Work out the finished part from the listing and answer in its coordinate system (mm). Round coordinates to 2 decimals unless told otherwise and drop trailing zeros. Loops run counter-clockwise (first coordinate to the right, second up) from the corner with the lowest first, then second, coordinate; pieces in that order, holes last. Notation, with made-up numbers: (61.25, 68.25) - (70.25, 68.25) arc R20 ccw to (70.25, 96.25) - close; hole circle Ø1 at (62.5, -13). An arc over 180 degrees is marked (long way). Answer as CSV lines item,"result". Start each with the question number.
```python
from build123d import *

# Parameters (mm, degrees)
F0_W     = 1016
F0_H     = 1930.4
F1_DEPTH = 50.8
F2_W     = 381
F2_H     = 304.8
F3_DEPTH = 50.801


with BuildPart() as f1:
    # F0 (on Front) → F1 (new body)
    with BuildSketch(Plane.XZ):
        Rectangle(F0_W, F0_H)
    extrude(amount=F1_DEPTH)

    # F2 (on face) → F3 (cut, through all)
    with BuildSketch(Plane.XZ.offset(50.8)):
        with Locations((-215.9, 660.4)):
            Rectangle(F2_W, F2_H)
        with Locations((-215.9, 330.2)):
            Rectangle(F2_W, F2_H)
        with Locations((-215.9, 0)):
            Rectangle(F2_W, F2_H)
        with Locations((-215.9, -330.2)):
            Rectangle(F2_W, F2_H)
        with Locations((-215.9, -660.4)):
            Rectangle(F2_W, F2_H)
        with Locations((215.9, 330.2)):
            Rectangle(F2_W, F2_H)
        with Locations((215.9, 660.4)):
            Rectangle(F2_W, F2_H)
        with Locations((215.9, 0)):
            Rectangle(F2_W, F2_H)
        with Locations((215.9, -330.2)):
            Rectangle(F2_W, F2_H)
        with Locations((215.9, -660.4)):
            Rectangle(F2_W, F2_H)
    extrude(amount=-F3_DEPTH, mode=Mode.SUBTRACT)


solid = f1.part
```
Item 1: Determine the mould class of faces 1 (the face through (-7, -25, 965.2)), 2 (the face through (508, -25, -14)), 3 (the face through (213, -26, -152.4)), 4 (the face through (-508, -25, -14)) for opening direction X: pulls with the +X half, pulls with the -X half, needs draft (parallel to the pull), parting line crosses it, or undercut.
Item 2: Section B-B, the plane x = 361 is taken. Give the vertices of the cut face in (y, z), and give its area (3 significant figures).
Item 3: Find the intervals of material crossed by L1, parallel to Z at x = 128.5, y = -33; L2, parallel to X at y = -12, z = -692, in increasing order.
Item 4: Section C-C, the plane y = -21.5 is taken. Count the separate pieces of the cut face and the enclosed holes in it, and give its area (3 significant figures).
Item 5: Section A-A, the plane z = 375.5 is taken. Give the vertices of the cut face in (x, y).
Answer:
1,face 1,"needs draft"
1,face 2,"pulls with the +X half"
1,face 3,"undercut"
1,face 4,"pulls with the -X half"
2,outline,"(-50.8, -965.2) - (0, -965.2) - (0, -812.8) - (-50.8, -812.8) - close; (-50.8, -508) - (0, -508) - (0, -482.6) - (-50.8, -482.6) - close; (-50.8, -177.8) - (0, -177.8) - (0, -152.4) - (-50.8, -152.4) - close; (-50.8, 152.4) - (0, 152.4) - (0, 177.8) - (-50.8, 177.8) - close; (-50.8, 482.6) - (0, 482.6) - (0, 508) - (-50.8, 508) - close; (-50.8, 812.8) - (0, 812.8) - (0, 965.2) - (-50.8, 965.2) - close"
2,area,"20,600 mm²"
3,L1,"z = -965.2 to -812.8, -508 to -482.6, -177.8 to -152.4, 152.4 to 177.8, 482.6 to 508, 812.8 to 965.2"
3,L2,"x = -508 to -406.4, -25.4 to 25.4, 406.4 to 508"
4,separate pieces,"1"
4,enclosed holes,"10"
4,area,"800,000 mm²"
5,outline,"(-508, -50.8) - (-406.4, -50.8) - (-406.4, 0) - (-508, 0) - close; (-25.4, -50.8) - (25.4, -50.8) - (25.4, 0) - (-25.4, 0) - close; (406.4, -50.8) - (508, -50.8) - (508, 0) - (406.4, 0) - close"
